Geometry: final body of the model. Coordinates: model frame, mm. Face numbers are marked on the shaded views. A direction names the side the tool comes from. Round coordinates to 2 decimals unless told otherwise and drop trailing zeros. Loops run counter-clockwise (first coordinate to the right, second up) from the corner with the lowest first, then second, coordinate; pieces in that order, holes last. Notation, with made-up numbers: (25.5, 2.5) - (32.5, 2.5) arc R11 ccw to (32.5, 17.5) - close; hole circle Ø3 at (-19.5, 81). An arc over 180 degrees is marked (long way). Answer as a JSON object with one key per item and string values. Group by question number.
Item 1: Line query: line 1 (X direction, y = 16.5, z = 41.5); line 2 (X direction, y = 5, z = 40.5); line 3 (Y direction, x = 7.5, z = 42). Output: solid intervals per line, ascending.
Item 2: Section A-A (y = 43). Return the cut outline in (x, z).
Item 3: Draft query along X for the marked faces 5, 6 and 7. Return one class per face: released by +X, released by -X, zero draft, split by the parting line, or undercut.
Item 4: First-contact query: pin 1 (12 mm diameter, centred on x = 22, y = 5.5, fed in from +Z); pin 2 (13 mm diameter, centred on x = 9, z = 0, fed in from -Y); pin 3 (13 mm diameter, centred on x = -30, y = 32, fed in from +Z). Flat tips, straight axial feed; report the tip coordinate or a pass-through.
Item 5: Reachability of the marked faces 1, 2, 3 and 4 from +Z, -Z, +X, -X, +Y, -Y: full face, straight path, thin tool, end or side. Return the list, or none.
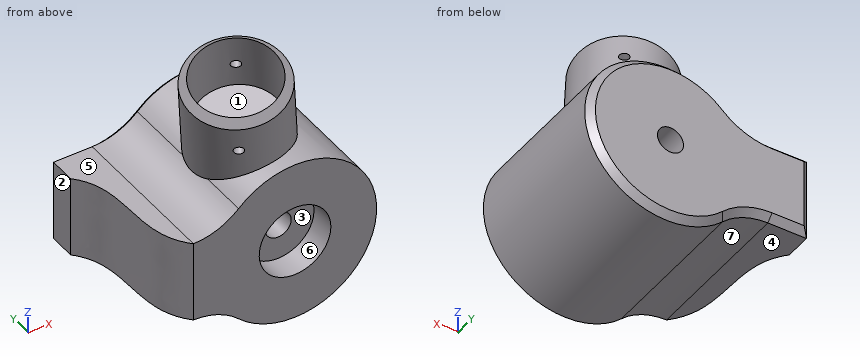
```python
from build123d import *

# Parameters (mm, degrees)
BOSS_EXTRUDE2_DEPTH = 50
CHAMFER1_SIZE       = 2
SKETCH3_R           = 15
BOSS_EXTRUDE3_DEPTH = 50
SKETCH5_R           = 12.7
CUT_EXTRUDE1_DEPTH  = 21
CHAMFER2_SIZE       = 3
SKETCH6_R           = 1.5
CUT_EXTRUDE2_DEPTH  = 48.5
SKETCH7_R           = 4
CUT_EXTRUDE3_DEPTH  = 82
SKETCH9_R           = 11
CUT_EXTRUDE4_DEPTH  = 8
CHAMFER3_SIZE       = 2
CUT_EXTRUDE5_DEPTH  = 96


with BuildPart() as part:
    # Sketch1 → Boss-Extrude2 (new body)
    with BuildSketch(Plane(origin=(0, 0, 0), x_dir=(1, 0, 0), z_dir=(0, 1, 0))):
        with BuildLine():
            Line((-34.047744375, -12.524843262), (-22.18855037, -12.524843262))
            ThreePointArc((-22.18855037, -12.524843262), (-14.720176785, -13.968492225), (-8.327835606, -18.091440268))
            ThreePointArc((-8.327835606, -18.091440268), (34.047744375, 0), (-8.327835606, 18.091440268))
            ThreePointArc((-8.327835606, 18.091440268), (-14.720176785, 13.968492225), (-22.18855037, 12.524843262))
            Line((-22.18855037, 12.524843262), (-34.047744375, 12.524843262))
            Line((-34.047744375, 12.524843262), (-34.047744375, -12.524843262))
        make_face()
    extrude(amount=BOSS_EXTRUDE2_DEPTH)

    # Chamfer1
    chamfer1_edges = [part.edges().sort_by_distance(p)[0] for p in [
        (-14.720176785, 50, 13.968492225),
        (34.047744375, 50, 0),
        (-14.720176785, 50, -13.968492225),
        (-28.118147372, 50, -12.524843262),
        (-28.118147372, 50, 12.524843262),
    ]]
    chamfer(chamfer1_edges, length=CHAMFER1_SIZE)

    # Sketch3 → Boss-Extrude3 (add)
    with BuildSketch(Plane(origin=(8.99805785, 25, 0), x_dir=(0.9847817818042102, -0.03725406297903357, 0.1697556391348433), z_dir=(-0.17379325152773012, -0.2062305980482824, 0.9629459206788651))):
        with Locations(Location((0, 0, 0), (0, 0, 159.473102118))):
            Circle(SKETCH3_R)
    extrude(amount=BOSS_EXTRUDE3_DEPTH)

    # Sketch5 → Cut-Extrude1 (cut)
    with BuildSketch(Plane(origin=(-7.521847234, -8.925749647, 41.676716708), x_dir=(0.9847817818042102, -0.03725406297903372, 0.16975563913484326), z_dir=(-0.17379325152773012, -0.2062305980482824, 0.9629459206788651))):
        with Locations(Location((7.929771868, 24.45263149, 0), (0, 0, 270.050317468))):
            Circle(SKETCH5_R)
    extrude(amount=-CUT_EXTRUDE1_DEPTH, mode=Mode.SUBTRACT)

    # Chamfer2
    # the kernel refuses this chamfer: 3 mm, written as the material it takes off along each edge
    with BuildSketch(Plane(origin=(0.308395273, 14.688470098, 48.147296034), x_dir=(-0.9219524467114961, 0.37774931122051036, -0.08549353118871512), z_dir=(0.3461207762127333, 0.9026485463906081, 0.255785085516762))) as chamfer2_piece_1:
        Polygon((15, -CHAMFER2_SIZE), (15 - CHAMFER2_SIZE, 0), (15, 0), align=None)
    revolve(axis=Axis((0.308395273, 14.688470098, 48.147296034), (-0.17379325152773012, -0.20623059804828237, 0.9629459206788651)), mode=Mode.SUBTRACT)

    # Sketch6 → Cut-Extrude2 (cut, symmetric)
    with BuildSketch(Plane(origin=(-22.18855037, 48, -12.524843262), x_dir=(-0.8657900557986787, 0.47372232177796453, 0.16122884707587404), z_dir=(-0.500365768548969, -0.82370873989167, -0.26671709635956337))):
        with Locations(Location((-27.977220625, -56.414440492, 0), (0, 0, 189.630227826))):
            Circle(SKETCH6_R)
    extrude(amount=CUT_EXTRUDE2_DEPTH, both=True, mode=Mode.SUBTRACT)

    # Sketch7 → Cut-Extrude3 (cut)
    with BuildSketch(Plane(origin=(0, 0, 0), x_dir=(-1, 0, 0), z_dir=(0, -1, 0))):
        with Locations(Location((-8.99805785, 0, 0), (0, 0, 90))):
            Circle(SKETCH7_R)
    extrude(amount=-CUT_EXTRUDE3_DEPTH, mode=Mode.SUBTRACT)

    # Sketch9 → Cut-Extrude4 (cut)
    with BuildSketch(Plane.XZ):
        with Locations(Location((8.99805785, 0, 0), (0, 0, 270))):
            Circle(SKETCH9_R)
    extrude(amount=-CUT_EXTRUDE4_DEPTH, mode=Mode.SUBTRACT)

    # Chamfer3
    chamfer3_edges = [part.edges().sort_by_distance(p)[0] for p in [
        (-34.047744375, 50, 0),
    ]]
    chamfer(chamfer3_edges, length=CHAMFER3_SIZE)

    # Sketch10 → Cut-Extrude5 (cut)
    with BuildSketch(Plane(origin=(0, 0, -12.524843262), x_dir=(-1, 0, 0), z_dir=(0, 0, -1))):
        with BuildLine():
            Line((22.186659572, 0), (34.047744375, 0))
            Line((34.047744375, 0), (34.047744375, 39.859182783))
            add(Edge.make_bspline(
                [(22.186659572, 0), (33.554101307, 11.263767606), (23.164669735, 28.934314706), (34.047744375, 39.859182783)],
                knots=[0, 0, 0, 0, 1, 1, 1, 1], degree=3))
        make_face()
    extrude(amount=-CUT_EXTRUDE5_DEPTH, mode=Mode.SUBTRACT)


solid = part.part
```
Values:
{
 "1": {"line 1": "x = -13.7 to -11.37, 14.41 to 16.75", "line 2": "x = -9 to -5.04, 7.58 to 11.54", "line 3": "y = 2.18 to 4.79, 27.68 to 30.29"},
 "2": {"outline": "(-34.05, -12.52) - (-22.19, -12.52) arc R20.04 cw to (-8.33, -18.09) arc R25.05 ccw (long way) to (-8.33, 18.09) arc R20.04 cw to (-22.19, 12.52) - (-34.05, 12.52) - close; hole circle Ø8 at (9, 0)"},
 "3": {"face 5": "zero draft", "face 6": "undercut", "face 7": "released by -X"},
 "4": {"pin 1": "stops at z = 24.05", "pin 2": "stops at y = 8", "pin 3": "stops at z = 12.52"},
 "5": {"face 1": "none", "face 2": "+Z, -Z, -X, +Y, -Y", "face 3": "-Y", "face 4": "-Z, -X, +Y, -Y"}
}
